from build123d import *

# Parameters (mm, degrees)
BOSS_EXTRUDE1_DEPTH    = 3.175
SKETCH3_W              = 20
SKETCH3_H              = 40
CUT_EXTRUDE1_DEPTH     = 131.03063341
M1_6_CLEARANCE_HOLE1_D = 1.7


with BuildPart() as part:
    # Sketch1 → Boss-Extrude1 (new body)
    with BuildSketch(Plane(origin=(0, 0, 0), x_dir=(1, 0, 0), z_dir=(0, 1, 0))):
        Polygon((-22.5, 0), (-22.5, 26.75), (22.5, 26.75), (22.5, 0), (28.85, 0), (28.85, -100), (22.5, -100), (22.5, -126.75), (-22.5, -126.75), (-22.5, -100), align=None)
    extrude(amount=BOSS_EXTRUDE1_DEPTH)

    # Sketch3 → Cut-Extrude1 (cut, through all)
    with BuildSketch(Plane(origin=(0, 3.175, 0), x_dir=(1, 0, 0), z_dir=(0, 1, 0))):
        with Locations((0, -94.9)):
            Rectangle(SKETCH3_W, SKETCH3_H)
    extrude(amount=-CUT_EXTRUDE1_DEPTH, mode=Mode.SUBTRACT)

    # M1.6 Clearance Hole1 (through all)
    with Locations(Plane(origin=(0, 3.175, 0), x_dir=(1, 0, 0), z_dir=(0, 1, 0))):
        with Locations((0, -70.4), (0, -119.4)):
            Hole(M1_6_CLEARANCE_HOLE1_D / 2)


solid = part.part
The listing builds one solid part. Answer for the finished solid, in the listing's coordinates (mm). A direction names the side the tool comes from. Round coordinates to 2 decimals unless told otherwise and drop trailing zeros. Write each loop counter-clockwise with the first axis right and the second up, starting at its lowest first coordinate (ties: lowest second). Pieces come first, ordered by that corner, then holes. Notation, with made-up numbers: (-36, 32.25) - (-12, 32.25) arc R21 ccw to (-12, 67.25) - close; hole circle Ø5 at (59.5, -8). An arc over 180 degrees is marked (long way). Use one line per item in the form item = value. Start each with the question number.
Item 1: Find the intervals of material crossed by line 1 (Z direction, x = 0, y = 0.9); line 2 (X direction, y = 0.9, z = 119.4); line 3 (X direction, y = 1.7, z = 70.4), in increasing order. Write a range as [from, to].
Item 2: A cutting plane is placed at B-B (y = 1.75). Write down the section's boundary in (x, z).
Item 3: A cutting plane is placed at A-A (x = -6). Write down the section's boundary in (y, z) (3 decimals), plus the area to 3 significant figures.
Item 4: Determine the mould class of faces 6 (the flat face through (22.5, 2, 113)), 7 (the flat face through (4, 0, 49)), 8 (the flat face through (0, 2, 114.9)), 9 (the flat face through (-10, 2, 95)) for opening direction X: +X half, -X half, draft (parallel to the pull), parting line (faces both ways), or undercut.
Item 5: Flat-ended cylindrical pins translate along their axes: pin 1 Ø5 at (x, z) = (-14, 110.5) entering from -Y; pin 2 Ø1 at (x, y) = (24.5, 1.5) entering from -Z; pin 3 Ø1.6 at (x, y) = (25, 2.5) entering from +Z; pin 4 Ø1.6 at (y, z) = (1.5, 118) entering from +X. Find the tip coordinate at first contact, or state that the pin passes through.
Item 6: A tool of negligible diameter and unlimited length cuts with its end or side. For faces 1 (the flat face through (26, 2, 100)), 2 (the flat face through (10, 2, 95)), 3 (the flat face through (4, 3.175, 49)), 4 (the flat face through (22.5, 2, -14)), 5 (the flat face through (-22.5, 2, 49)), from which of +Z, -Z, +X, -X, +Y, -Y can it reach the whole face along a straight path? Write none if from no direction.
The answers:
q1.line_1 = [-26.75, 69.55], [71.25, 74.9], [114.9, 118.55], [120.25, 126.75]
q1.line_2 = [-22.5, -0.85], [0.85, 22.5]
q1.line_3 = [-22.5, -0.85], [0.85, 28.85]
q2.outline = (-22.5, -26.75) - (22.5, -26.75) - (22.5, 0) - (28.85, 0) - (28.85, 100) - (22.5, 100) - (22.5, 126.75) - (-22.5, 126.75) - close; hole (-10, 74.9) - (10, 74.9) - (10, 114.9) - (-10, 114.9) - close; hole circle Ø1.7 at (0, 70.4); hole circle Ø1.7 at (0, 119.4)
q3.outline = (0, -26.75) - (3.175, -26.75) - (3.175, 74.9) - (0, 74.9) - close; (0, 114.9) - (3.175, 114.9) - (3.175, 126.75) - (0, 126.75) - close
q3.area = 360 mm^2
q4.face_6 = +X half
q4.face_7 = draft
q4.face_8 = undercut
q4.face_9 = undercut
q5.pin_1 = 0
q5.pin_2 = 0
q5.pin_3 = 100
q5.pin_4 = 22.5
q6.face_1 = +Z, +X, +Y, -Y
q6.face_2 = +Y, -Y
q6.face_3 = +Z, -Z, +X, -X, +Y
q6.face_4 = -Z, +X, +Y, -Y
q6.face_5 = +Z, -Z, -X, +Y, -Y
